Autodesk Fusion 360 part; units mm, degrees
sketch "Sketch1" plane through (0, 0, 0) normal (0, 0, 1) x (1, 0, 0)
  line L0 (11.5304, 55) -> (-0.0094, 35)
  line L1 (-0.0094, 35) -> (0, 0)
  line L2 (0, 0) -> (6.0773, -10.5197)
  line L3 (17.8607, -11.0501) -> (25.6471, 0)
  line L4 (15.8612, 52.5012) -> (4.9909, 33.6616)
  line L5 (4.9909, 33.6616) -> (4.9996, 1.3411)
  line L6 (4.9996, 1.3411) -> (8.0596, -3.9556)
  line L7 (16.4762, -4.3344) -> (21.5599, 2.88)
  line L8 (11.5304, 55) -> (15.8612, 52.5012)
  line L9 (25.6471, 0) -> (21.5599, 2.88)
  arc A0 (8.0596, -3.9556) -> (16.4762, -4.3344) centre (12.389, -1.4544) ccw
  arc A1 (6.0773, -10.5197) -> (17.8607, -11.0501) centre (12.1386, -7.0181) ccw
  point P0 (11.5542, -20)
  dimension "d16" = 35
  dimension "d17" = 150
  dimension "d18" = 150
  dimension "d19" = 20
  dimension "d20" = 20
  dimension "d21" = 20
  dimension "d23" = 5
  dimension "d24" = 7
extrude "Extrude1" add sketch "Sketch1" along normal blind 15
sketch "Sketch2" plane through (5, 0.0013, 0) normal (1, 0.0003, 0) x (0, 0, -1)
  line L0 (0, 1.3397) -> (0, 33.6603)
  line L1 (0, 33.6603) -> (-15, 33.6603)
  line L2 (-15, 33.6603) -> (-15, 1.3397)
  line L3 (-15, 1.3397) -> (0, 1.3397)
  line L4 (-7.5, 33.6603) -> (-7.5, 1.3397) construction
  line L5 (0, 17.5) -> (-15, 17.5) construction
  circle A0 centre (-7.5, 25.6603) radius 4
  circle A1 centre (-7.5, 9.3397) radius 4
  dimension "d27" = 8
  dimension "d28" = 8
extrude "Extrude2" cut sketch "Sketch2" against normal blind 3 draft -35 contours A0 | A1
extrude "Extrude3" cut 2 faces at (1.9929, 26.1558, 7.387) (1.9973, 9.8353, 7.0106) along direction (-1, -0.00027, 0) through all
fillet "Fillet1" radius 7.5 4 edges at (13.6958, 53.7506, 15) (13.6958, 53.7506, 0) (23.6035, 1.44, 15) (23.6035, 1.44, 0)
fillet "Fillet2" radius 8 2 edges at (-0.0094, 35, 7.5) (0, 0, 7.5)
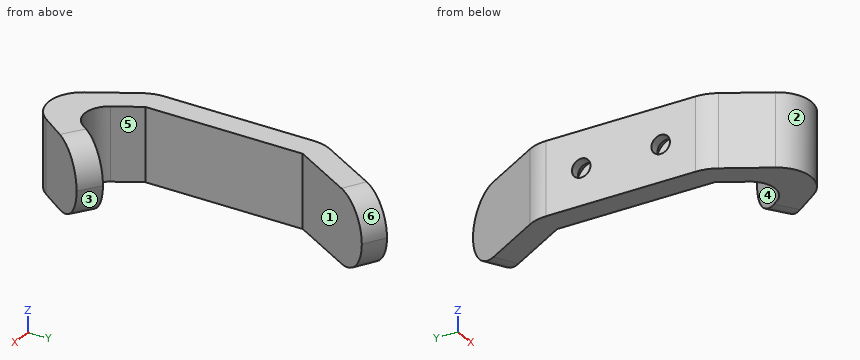
The model under review builds one solid part; all positions refer to its coordinate system, in mm. Face numbers are marked on the shaded views. A direction names the side the tool comes from. Give positions to 0.01 mm unless a question says otherwise; leave off trailing zeros. Order: outer loops, then holes, each group sorted by start corner. A loop starts at its lowest first (then second) coordinate and runs counter-clockwise, first axis right, second up. Notation, with made-up numbers: M 40,83 L 77,83 A31 cw 77,112 Z; hole C -7,-37 d4. An arc over 180 degrees is marked long. One line per question, with ' | ' between items. Start each with the question number.
1) Clearance check with flat-ended pins moving along their axes: P1, Ø1, axis at x = 5.5, z = 11.5, coming from the +Y side; P2, Ø1.5, axis at y = 9, z = 3, coming from the +X side; P3, Ø3, axis at x = 6, y = 27, coming from the +Z side; P4, Ø6, axis at x = 8, z = 6.5, coming from the +Y side. State where each tip first meets the part, or that it passes through.
2) Wall thickness on L1, parallel to Y at x = 2, z = 8.25; L2, parallel to X at y = 9, z = 12.25; L3, parallel to Z at x = 21, y = -5.5: over which ranges is each line inside the solid? List them lowest first. Write a range as from..to.
3) Consider section A-A, the plane x = 3.25. State how many separate pieces and enclosed holes the cut face has, then the cut area to 3 significant figures.
4) For the marked faces 4, 5 and 6, list the 3-axis set-ups (+Z, -Z, +X, -X, +Y, -Y) from which the entire face can be reached by the end or side of a thin tool; tool diameter is ignored.
5) Consider section B-B, the plane y = 18. Give the boundary of the cut face in (x, z).
6) Mouldability with a two-part tool opening along Y and no side actions: class the marked faces 1, 2 and 3 as pulls with the +Y half, pulls with the -Y half, needs draft (parallel to the pull), parting line crosses it, or undercut.
Found:
1) P1: stops at y = 45.42 | P2: stops at x = 5 | P3: stops at z = 15 | P4: stops at y = 54.08
2) L1: y = -3.46..7.59, 11.09..23.91, 27.41..38.48 | L2: x = 0..5 | L3: z = 0.01..14.99
3) separate pieces: 1 | enclosed holes: 2 | area: 646 mm²
4) face 4: +Z, -Z, +Y | face 5: +Z, -Z | face 6: +Z, +X, +Y
5) outline: M 0,0 L 5,0 L 5,15 L 0,15 Z
6) face 1: undercut | face 2: pulls with the -Y half | face 3: pulls with the +Y half
